Read the model definition and answer for the solid it produces. Units are mm, in the model's axes. Coordinates: 2 decimals unless noted, no trailing zeros. Loops run counter-clockwise (first coordinate to the right, second up) from the corner with the lowest first, then second, coordinate; pieces in that order, holes last. Notation, with made-up numbers: M -25,61.5 L -9,61.5 A20 ccw -9,98.5 Z; hole C -28.5,-40 d11. An arc over 180 degrees is marked long. Put each result on its own line as item: value.
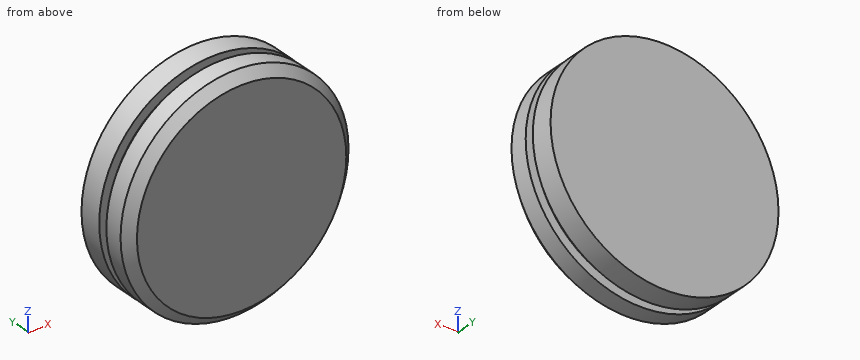
Autodesk Inventor part; units mm, degrees
ref_plane "YZ Plane" through (0, 0, 0) normal (1, 0, 0) x (0, 1, 0)
ref_plane "XZ Plane" through (0, 0, 0) normal (0, 1, 0) x (-1, 0, 0)
ref_plane "XY Plane" through (0, 0, 0) normal (0, 0, 1) x (1, 0, 0)
sketch "Sketch1" plane through (0, 0, 0) normal (0, 0, 1) x (1, 0, 0)
  line L0 (0, 0) -> (-22.5, 0)
  line L1 (-24.5, 13) -> (0, 13)
  line L2 (0, 13) -> (0, 0)
  line L3 (-22.5, 0) -> (-24.5, 2)
  line L4 (-24.5, 8) -> (-22.5, 8)
  line L5 (-22.5, 8) -> (-22.5, 6)
  line L6 (-22.5, 6) -> (-24.5, 6)
  line L7 (-24.5, 6) -> (-24.5, 8)
  line L8 (-24.5, 2) -> (-24.5, 6)
  line L9 (-24.5, 8) -> (-24.5, 13)
  point P0 (-24.5, 0)
  dimension "d0" = 24.5
  dimension "d1" = 13
  dimension "d2" = 2
  dimension "d3" = 2
  dimension "d4" = 2
  dimension "d5" = 2
  dimension "d6" = 5
  dimension "d7" = 45
revolve "Revolution1" add sketch "Sketch1" angle 360 about axis through (0, 13, 0) along (0, -1, 0) contours L0 L3 L8 L6 L5 L4 L9 L1 L2
properties part number "bulkhead"
1) Find section C-C, the plane y = 9.25. Write down the section's boundary in (x, z), plus the area to 3 significant figures.
Answer list:
outline: C 0,0 d49
area: 1,890 mm^2
2) Straight lines are drawn through the part: line 1 (Y direction, x = -20.5, z = 10); line 2 (X direction, y = 6.75, z = -18); line 3 (Z direction, x = 4.5, y = 10.5). For each, find the intervals that lie inside material, in ascending order. Write a range as [from, to].
Answer list:
line 1: y = [0.31, 6], [8, 13]
line 2: x = [-13.5, 13.5]
line 3: z = [-24.08, 24.08]
3) Find section B-B, the plane z = 0. Write down the section's boundary in (x, y).
Answer list:
outline: M -24.5,2 L -22.5,0 L 22.5,0 L 24.5,2 L 24.5,6 L 22.5,6 L 22.5,8 L 24.5,8 L 24.5,13 L -24.5,13 L -24.5,8 L -22.5,8 L -22.5,6 L -24.5,6 Z
4) Find section A-A, the plane x = 0. Write down the section's boundary in (y, z).
Answer list:
outline: M 0,-22.5 L 2,-24.5 L 6,-24.5 L 6,-22.5 L 8,-22.5 L 8,-24.5 L 13,-24.5 L 13,24.5 L 8,24.5 L 8,22.5 L 6,22.5 L 6,24.5 L 2,24.5 L 0,22.5 Z
5) Given pin 1 Ø4 at (y, z) = (11, -5.5) entering from +X; pin 2 Ø4 at (x, y) = (-0.5, 8) entering from +Z; pin 3 Ø1.5 at (y, z) = (2, -3.5) entering from -X, each flat-ended and moving along its own axis, determine where each tip first touches the part or whether it passes through.
Answer list:
pin 1: stops at x = 24.25
pin 2: stops at z = 24.5
pin 3: stops at x = -24.35
